```python
from build123d import *

# Parameters (mm, degrees)
PLAT_W                      = 50
PLAT_H                      = 5
EL_MENT_M_CANO_SOUD_1_DEPTH = 470
ESQUISSE7_W                 = 30
ESQUISSE7_H                 = 25
ENL_V_MAT_EXTRU_2_DEPTH     = 6
R_P_TITION_LIN_AIRE2_COUNT  = 8
R_P_TITION_LIN_AIRE2_PITCH  = 56
ESQUISSE8_R                 = 5.5
ENL_V_MAT_EXTRU_3_DEPTH     = 5
R_P_TITION_LIN_AIRE3_COUNT  = 4
R_P_TITION_LIN_AIRE3_PITCH  = 146.6


with BuildPart() as part:
    # plat → Elément mécano-soudé1 (new body)
    with BuildSketch(Plane.YZ.offset(-235)):
        Rectangle(PLAT_W, PLAT_H)
    extrude(amount=EL_MENT_M_CANO_SOUD_1_DEPTH)

    # Esquisse7 → Enlèv. mat.-Extru.2 (cut, through all)
    with BuildSketch(Plane.XY.offset(2.5)):
        with Locations((-195, 12.5)):
            Rectangle(ESQUISSE7_W, ESQUISSE7_H)
    enl_v_mat_extru_2 = extrude(amount=-ENL_V_MAT_EXTRU_2_DEPTH, mode=Mode.SUBTRACT)

    # Répétition linéaire2: Enlèv. mat.-Extru.2 ×8
    with Locations(*[(i * R_P_TITION_LIN_AIRE2_PITCH, 0, 0) for i in range(1, R_P_TITION_LIN_AIRE2_COUNT)]):
        add(enl_v_mat_extru_2, mode=Mode.SUBTRACT)

    # Esquisse8 → Enlèv. mat.-Extru.3 (cut, symmetric)
    with BuildSketch(Plane.XY):
        with Locations((-220, -13)):
            Circle(ESQUISSE8_R)
    enl_v_mat_extru_3 = extrude(amount=ENL_V_MAT_EXTRU_3_DEPTH, both=True, mode=Mode.SUBTRACT)

    # Répétition linéaire3: Enlèv. mat.-Extru.3 ×4
    with Locations(*[(i * R_P_TITION_LIN_AIRE3_PITCH, 0, 0) for i in range(1, R_P_TITION_LIN_AIRE3_COUNT)]):
        add(enl_v_mat_extru_3, mode=Mode.SUBTRACT)


solid = part.part
```
Geometry: final body of the model. Coordinates: model frame, mm. Round coordinates to 2 decimals unless told otherwise and drop trailing zeros. Order: outer loops, then holes, each group sorted by start corner. A loop starts at its lowest first (then second) coordinate and runs counter-clockwise, first axis right, second up. Notation, with made-up numbers: M -31,87.5 L 5,87.5 A25 cw 5,113.5 Z; hole C 28,68.25 d7. An arc over 180 degrees is marked long. Use one line per item in the form item = value. Start each with the question number.
Q1. Cut plane A-A (x = -220). Return loops of the section in (y, z), and give its area (3 significant figures).
Q2. Cut plane C-C (x = -73.4). Return loops of the section in (y, z), and give its area (3 significant figures).
Q3. Cut plane B-B (z = 0.15). Count the separate pieces of the cut face and the enclosed holes in it, and give its area (3 significant figures).
Q4. Material intervals for line 1 (X direction, y = -12, z = -0.8); line 2 (Y direction, x = 219.8, z = -0.4); line 3 (Y direction, x = 73.2, z = 0.9), sorted ascending. Write a range as [from, to].
Q5. Pin query (flat end, axial travel): pin 1 Ø2.5 at (x, z) = (82.5, 0.5) entering from +Y. Return the tip coordinate at first contact, or that it passes through.
Q6. Mould query, pull axis X, two halves, no side actions, for faces 1 (the face through (-3, 0, 2.5)), 2 (the face through (-225.495, -12.758, 0.035)). Classes: +X half, -X half, draft (parallel to the pull), parting line (faces both ways), or undercut.
Geometry results:
q1.outline = M -25,-2.5 L -18.5,-2.5 L -18.5,2.5 L -25,2.5 Z; M -7.5,-2.5 L 25,-2.5 L 25,2.5 L -7.5,2.5 Z
q1.area = 195 mm^2
q2.outline = M -25,-2.5 L -18.5,-2.5 L -18.5,2.5 L -25,2.5 Z; M -7.5,-2.5 L 0,-2.5 L 0,2.5 L -7.5,2.5 Z
q2.area = 70.0 mm^2
q3.separate_pieces = 1
q3.enclosed_holes = 4
q3.area = 17,100 mm^2
q4.line_1 = [-235, -225.41], [-214.59, -78.81], [-67.99, 67.79], [78.61, 214.39], [225.21, 235]
q4.line_2 = [-25, -18.5], [-7.5, 25]
q4.line_3 = [-25, -18.5], [-7.5, 0]
q5.pin_1 = 0
q6.face_1 = draft
q6.face_2 = undercut
